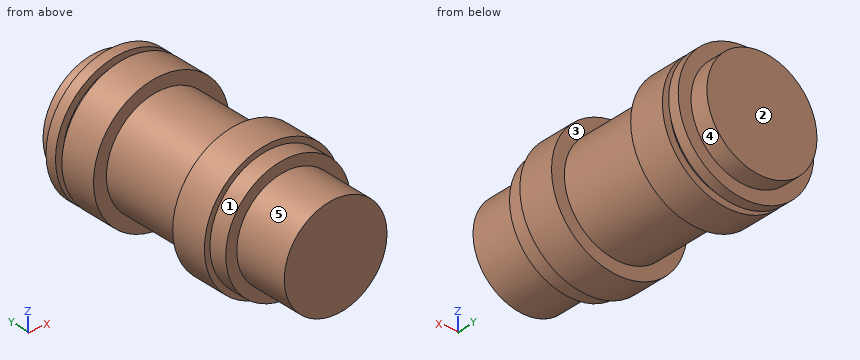
from build123d import *

# Parameters (mm, degrees)
F0_R      = 17
F1_DEPTH  = 5
F2_R      = 14
F3_DEPTH  = 15
F4_R      = 18.5
F5_DEPTH  = 10
F6_R      = 15
F7_DEPTH  = 35
F8_R      = 18.5
F9_DEPTH  = 10
F10_R     = 16.5
F11_DEPTH = 2
F12_R     = 18.5
F13_DEPTH = 3
F14_R     = 15
F15_DEPTH = 5


with BuildPart() as f1:
    # F0 (on Front) → F1 (new body)
    with BuildSketch(Plane.XZ):
        Circle(F0_R)
    extrude(amount=F1_DEPTH)

    # F2 (on face) → F3 (join)
    with BuildSketch(Plane.XZ.offset(5)):
        Circle(F2_R)
    extrude(amount=F3_DEPTH)

    # F4 (on Front) → F5 (join)
    with BuildSketch(Plane.XZ):
        Circle(F4_R)
    extrude(amount=-F5_DEPTH)

    # F6 (on Front) → F7 (join)
    with BuildSketch(Plane.XZ):
        Circle(F6_R)
    extrude(amount=-F7_DEPTH)

    # F8 (on face) → F9 (join)
    with BuildSketch(Plane(origin=(0, 35, 0), x_dir=(-1, 0, 0), z_dir=(0, 1, 0))):
        Circle(F8_R)
    extrude(amount=F9_DEPTH)

    # F10 (on face) → F11 (join)
    with BuildSketch(Plane(origin=(0, 45, 0), x_dir=(-1, 0, 0), z_dir=(0, 1, 0))):
        Circle(F10_R)
    extrude(amount=F11_DEPTH)

    # F12 (on face) → F13 (join)
    with BuildSketch(Plane(origin=(0, 47, 0), x_dir=(-1, 0, 0), z_dir=(0, 1, 0))):
        Circle(F12_R)
    extrude(amount=F13_DEPTH)

    # F14 (on face) → F15 (join)
    with BuildSketch(Plane(origin=(0, 50, 0), x_dir=(-1, 0, 0), z_dir=(0, 1, 0))):
        Circle(F14_R)
    extrude(amount=F15_DEPTH)


solid = f1.part
Source: CAD feature listing. Evaluate the final solid. Frame: model axes, mm. Face numbers are marked on the shaded views. A direction names the side the tool comes from. Coordinates: 2 decimals unless noted, no trailing zeros. Loops run counter-clockwise (first coordinate to the right, second up) from the corner with the lowest first, then second, coordinate; pieces in that order, holes last. Notation, with made-up numbers: (72.25, 32) - (109.25, 32) arc R26 cw to (109.25, 48) - close; hole circle Ø2 at (-3, 55). An arc over 180 degrees is marked (long way). One line per item, written item: value. Start each with the question number.
1. Section C-C (y = 19.5). Return the cut outline in (x, z).
2. Section D-D (y = 2). Return the cut outline in (x, z).
3. Set-up query: the marked faces 3, 4 and 5. Return all of +Z, -Z, +X, -X, +Y, -Y with unobstructed straight access to the full face (end or side cutting, diameter ignored); none if empty.
4. Ray query, L1, parallel to Y at x = 16.5, z = -3.5; L2, parallel to Y at x = -8.5, z = 15.5; L3, parallel to Y at x = 1.5, z = -15. Return the intervals inside material, ascending.
5. Contact query for flat-ended pins moving along their axis: P1, Ø3, axis at x = -6, y = 9.5, coming from the +Z side; P2, Ø2, axis at y = 15, z = 8.5, coming from the -X side; P3, Ø1, axis at y = 6, z = 4, coming from the +X side. Output: stop coordinate, or through.
6. Mould query, pull axis X, two halves, no side actions, for the marked faces 1 and 2. Classes: pulls with the +X half, pulls with the -X half, needs draft (parallel to the pull), parting line crosses it, or undercut.
Verdict:
1. outline: circle Ø30 at (0, 0)
2. outline: circle Ø37 at (0, 0)
3. face 3: none
3. face 4: +Y
3. face 5: -Y
4. L1: y = -5 to 10, 35 to 45, 47 to 50
4. L2: y = 0 to 10, 35 to 45, 47 to 50
4. L3: y = -5 to 10, 35 to 50
5. P1: stops at z = 17.94
5. P2: stops at x = -12.99
5. P3: stops at x = 18.17
6. face 1: parting line crosses it
6. face 2: needs draft
